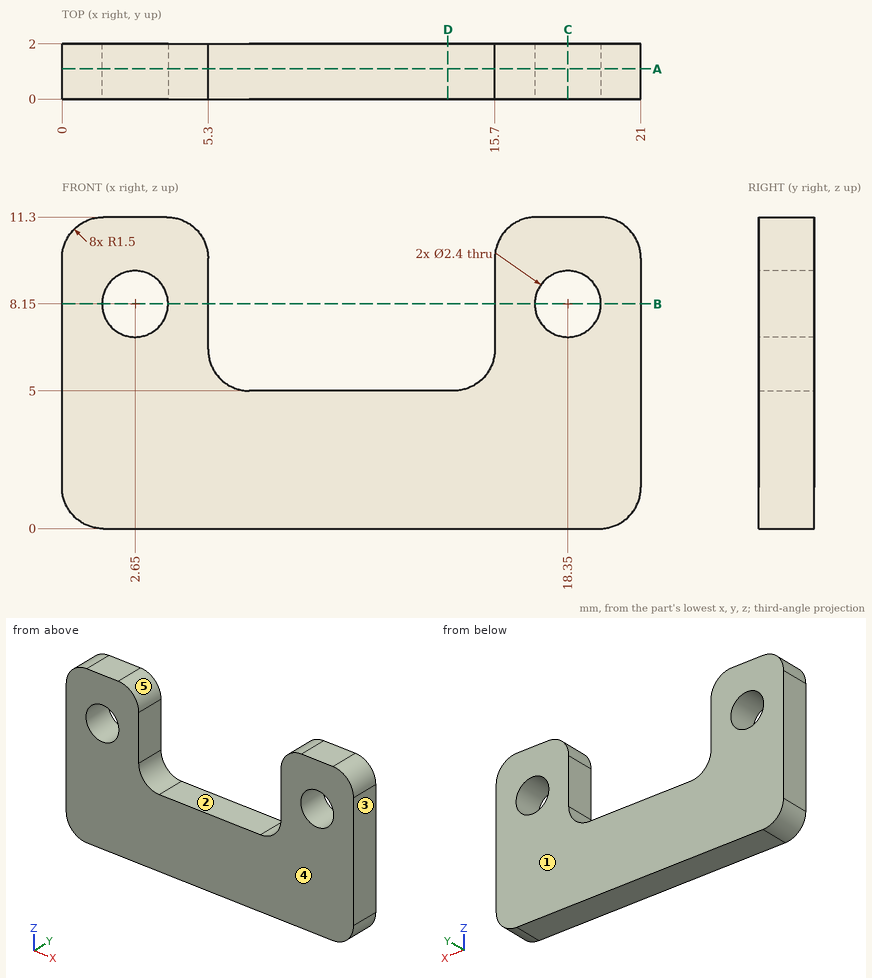
For this review, use the dimensioned drawing (mm, ordinates from the lowest corner) and the shaded views. A direction names the side the tool comes from. Round coordinates to 2 decimals unless told otherwise and drop trailing zeros. Write each loop counter-clockwise with the first axis right and the second up, starting at its lowest first coordinate (ties: lowest second). Pieces come first, ordered by that corner, then holes. Notation, with made-up numbers: (57.5, -27) - (83.5, -27) arc R23 cw to (83.5, -8) - close; hole circle Ø11 at (60, 58). An arc over 180 degrees is marked (long way). Answer as CSV lines item,"result". Start each with the question number.
(1) We need section A-A on y = 1.1. State the section outline as (x, z) points, plus the area to 3 significant figures.
(2) To check wall thickness, follow line 1 (X direction, y = 0.65, z = 8.15); line 2 (Z direction, x = 2.65, y = 0.9); line 3 (X direction, y = 1.25, z = 6.5). State the ranges of each line that lie inside material, in increasing order.
(3) We need section B-B on z = 8.15. State the section outline as (x, y) points, plus the area to 3 significant figures.
(4) For pin 1 Ø1.9 at (x, z) = (18.35, 8.15) entering from +Y, flat-tipped, find the tip position at first contact; note if it passes through.
(5) For the marked faces 4 and 5, list the 3-axis set-ups (+Z, -Z, +X, -X, +Y, -Y) from which the entire face can be reached by the end or side of a thin tool; tool diameter is ignored.
(6) We need section C-C on x = 18.35. State the section outline as (y, z) points, plus the area to 3 significant figures.
(7) We need section D-D on x = 14. State the section outline as (y, z) points.
(8) Draft analysis for pull direction X (two halves, no side actions). For the marked faces 1, 2 and 3, state which applies: pulls with the +X half, pulls with the -X half, needs draft (parallel to the pull), parting line crosses it, or undercut.
Worked answers:
1,outline,"(0, 1.5) arc R1.5 ccw to (1.5, 0) - (19.5, 0) arc R1.5 ccw to (21, 1.5) - (21, 9.8) arc R1.5 ccw to (19.5, 11.3) - (17.2, 11.3) arc R1.5 ccw to (15.7, 9.8) - (15.7, 6.5) arc R1.5 cw to (14.2, 5) - (6.8, 5) arc R1.5 cw to (5.3, 6.5) - (5.3, 9.8) arc R1.5 ccw to (3.8, 11.3) - (1.5, 11.3) arc R1.5 ccw to (0, 9.8) - close; hole circle Ø2.4 at (2.65, 8.15); hole circle Ø2.4 at (18.35, 8.15)"
1,area,"161 mm²"
2,line 1,"0 to 1.45, 3.85 to 5.3, 15.7 to 17.15, 19.55 to 21"
2,line 2,"0 to 6.95, 9.35 to 11.3"
2,line 3,"0 to 5.3, 15.7 to 21"
3,outline,"(0, 0) - (1.45, 0) - (1.45, 2) - (0, 2) - close; (3.85, 0) - (5.3, 0) - (5.3, 2) - (3.85, 2) - close; (15.7, 0) - (17.15, 0) - (17.15, 2) - (15.7, 2) - close; (19.55, 0) - (21, 0) - (21, 2) - (19.55, 2) - close"
3,area,"11.6 mm²"
4,pin 1,"through"
5,face 4,"+Z, -Z, +X, -X, -Y"
5,face 5,"+Z, +Y, -Y"
6,outline,"(0, 0) - (2, 0) - (2, 6.95) - (0, 6.95) - close; (0, 9.35) - (2, 9.35) - (2, 11.3) - (0, 11.3) - close"
6,area,"17.8 mm²"
7,outline,"(0, 0) - (2, 0) - (2, 5) - (0, 5) - close"
8,face 1,"needs draft"
8,face 2,"undercut"
8,face 3,"pulls with the +X half"
